from build123d import *

# Parameters (mm, degrees)
F1_DEPTH       = 1121.496
F3_DEPTH       = 304.801
F6_D           = 9
F6_DEPTH       = 10
F6_CBORE_D     = 12
F6_CBORE_DEPTH = 1.5
F8_DEPTH       = 304.8


with BuildPart() as f1:
    # F0 (on Front) → F1 (new body)
    with BuildSketch(Plane.XZ):
        with BuildLine():
            Line((-66.6495, -50.8), (-9.5504, -50.8))
            ThreePointArc((-9.5504, -50.8), (-2.797247, -48.002753), (0, -41.2496))
            Line((0, -41.2496), (0, 244.4495))
            ThreePointArc((0, 244.4495), (-2.797277, 251.202723), (-9.5505, 254))
            Line((-9.5505, 254), (-66.6496, 254))
            ThreePointArc((-66.6496, 254), (-73.402753, 251.202753), (-76.2, 244.4496))
            Line((-76.2, 244.4496), (-76.2, -41.2495))
            ThreePointArc((-76.2, -41.2495), (-73.402723, -48.002723), (-66.6495, -50.8))
        make_face()
        with BuildLine():
            ThreePointArc((-71.4248, 244.4496), (-70.026176, 247.826176), (-66.6496, 249.2248))
            Line((-66.6496, 249.2248), (-9.5504, 249.2248))
            ThreePointArc((-9.5504, 249.2248), (-6.173824, 247.826176), (-4.7752, 244.4496))
            Line((-4.7752, 244.4496), (-4.7752, -41.2496))
            ThreePointArc((-4.7752, -41.2496), (-6.173824, -44.626176), (-9.5504, -46.0248))
            Line((-9.5504, -46.0248), (-66.6496, -46.0248))
            ThreePointArc((-66.6496, -46.0248), (-70.026176, -44.626176), (-71.4248, -41.2496))
            Line((-71.4248, -41.2496), (-71.4248, 244.4496))
        make_face(mode=Mode.SUBTRACT)
    extrude(amount=F1_DEPTH)

    # F2 (on face) → F3 (cut, through all)
    with BuildSketch(Plane.XY.offset(254)):
        Polygon((0, 0), (-76.2, 0), (0, -76.2), align=None)
        Polygon((0, -1045.296), (-76.2, -1121.496), (0, -1121.496), align=None)
    extrude(amount=-F3_DEPTH, mode=Mode.SUBTRACT)


with BuildPart() as f1_1:
    # F4: moved
    add(f1.part.moved(Location((0, 25.4, 0))))

    # F6
    with Locations(Plane.YZ):
        with Locations((-892.429, 165.784009), (-892.429, 122.784009), (-892.429, 79.784009), (-892.429, 36.784009), (-892.429, -6.215991), (-607.3902, 165.784009), (-607.3902, 122.784009), (-607.3902, 79.784009), (-607.3902, 36.784009), (-607.3902, -6.215991), (-399.8468, 165.784009), (-399.8468, 122.784009), (-399.8468, 79.784009), (-399.8468, 36.784009), (-399.8468, -6.215991), (-114.808, 165.784009), (-114.808, 122.784009), (-114.808, 79.784009), (-114.808, 36.784009), (-114.808, -6.215991)):
            CounterBoreHole(F6_D / 2, F6_CBORE_D / 2, F6_CBORE_DEPTH, depth=F6_DEPTH)

    # F7 (on face) → F8 (cut, through all)
    with BuildSketch(Plane.XY.offset(254)):
        Polygon((0, -952.008), (-76.2, -1028.208), (-76.2, -1096.096), (0, -1096.096), align=None)
    extrude(amount=-F8_DEPTH, mode=Mode.SUBTRACT)


solid = f1_1.part
Model file for the job. Use its own axes, mm. A direction names the side the tool comes from. Coordinates: 2 decimals unless noted, no trailing zeros. Write each loop counter-clockwise with the first axis right and the second up, starting at its lowest first coordinate (ties: lowest second). Pieces come first, ordered by that corner, then holes. Notation, with made-up numbers: (75, -0.75) - (88, -0.75) arc R31 cw to (88, 28.25) - close; hole circle Ø11 at (35.25, 2.5). An arc over 180 degrees is marked (long way). Write each question's results on one line, items separated by ' | '. Start each with the question number.
1) Cut at A-A (z = 19). Write the cut outline in (x, y).
2) Probe line 1 along X through (y, z) = (-388.5, 156); line 2 along Z through (x, y) = (-36, -916.5); line 3 along X through (y, z) = (-27, 44). List the from-to ranges inside material, lowest first. Write a range as from..to.
3) Mould opens along Z. For faces 1 (the face through (-38, -494, -50.8)), 2 (the face through (-4.775, -495, 104)), 3 (the face through (-76.2, -494, 104)) say: pulls with the +Z half, pulls with the -Z half, needs draft (parallel to the pull), parting line crosses it, or undercut.
4) 3-axis set-ups, long thin cutter, end or side, ignore diameter. For faces 4 (the face through (-71.425, -494, 100)), 5 (the face through (-4.056, -956.064, 102.311)): which of +Z, -Z, +X, -X, +Y, -Y reach the whole face in a straight line?
5) Cut at C-C (x = -39). Write the cut outline in (y, z), then the cut area to 3 significant figures.
6) Flat gauge pins, fed straight in: P1, Ø11, axis at y = -607.39, z = 165.78, coming from the +X side; P2, Ø3.5, axis at y = -892, z = 166, coming from the +X side. Where does each tip first touch, or does it go through?
7) Cut at B-B (y = -671.5). Write the cut outline in (x, z).
Returned:
1) outline: (-76.2, -1028.21) - (-71.42, -1023.43) - (-71.42, 20.62) - (-76.2, 25.4) - close; (-4.78, -956.78) - (0, -952.01) - (0, -50.8) - (-4.78, -46.02) - close
2) line 1: -76.2..-71.42, -4.78..0 | line 2: -50.8..-46.02, 249.22..254 | line 3: -76.2..-71.42
3) face 1: pulls with the -Z half | face 2: undercut | face 3: needs draft
4) face 4: +Y, -Y | face 5: +Z, -Z, +X, -Y
5) outline: (-991.01, -50.8) - (-11.8, -50.8) - (-11.8, -46.02) - (-991.01, -46.02) - close; (-991.01, 249.22) - (-11.8, 249.22) - (-11.8, 254) - (-991.01, 254) - close | area: 9,350 mm^2
6) P1: x = -1.5 | P2: x = -71.42
7) outline: (-76.2, -41.25) arc R9.55 ccw to (-66.65, -50.8) - (-9.55, -50.8) arc R9.55 ccw to (0, -41.25) - (0, 244.45) arc R9.55 ccw to (-9.55, 254) - (-66.65, 254) arc R9.55 ccw to (-76.2, 244.45) - close; hole (-71.42, -41.25) arc R4.78 ccw to (-66.65, -46.02) - (-9.55, -46.02) arc R4.78 ccw to (-4.78, -41.25) - (-4.78, 244.45) arc R4.78 ccw to (-9.55, 249.22) - (-66.65, 249.22) arc R4.78 ccw to (-71.42, 244.45) - close
